Part model, mm, in its own coordinate system. A direction names the side the tool comes from. Give positions to 0.01 mm unless a question says otherwise; leave off trailing zeros. Write each loop counter-clockwise with the first axis right and the second up, starting at its lowest first coordinate (ties: lowest second). Pieces come first, ordered by that corner, then holes. Notation, with made-up numbers: M -16.5,57.5 L 20.5,57.5 A32 ccw 20.5,87.5 Z; hole C 7.5,50 d7. An arc over 180 degrees is marked long. Answer as CSV lines item,"result". Start each with the question number.
Item 1: Pin check, flat tips, straight feed: pin 1 (2.5 mm diameter, centred on y = 3, z = 11, fed in from -X); pin 2 (5 mm diameter, centred on x = -17.5, z = 24, fed in from +Y); pin 3 (1.5 mm diameter, centred on y = 18, z = 27.5, fed in from +X). Stop position of each tip, or through.
Item 2: Wall check: L1, parallel to Y at x = -9.25, z = 26.5; L2, parallel to X at y = 10, z = 28.5. Give the ranges that are in metal, low to high. Write a range as from..to.
Item 3: 3-axis set-ups, long thin cutter, end or side, ignore diameter. For faces 1 (the flat face through (-23, 30, 27)), 2 (the flat face through (-21, 8, 25)), 3 (the flat face through (-20, 17, 27)): which of +Z, -Z, +X, -X, +Y, -Y reach the whole face in a straight line?
Item 4: Band-saw the part on B-B, the plane z = 14. List the corners of the cut face in (x, y).
Item 5: Band-saw the part on C-C, the plane x = -4.5. List the corners of the cut face in (y, z).
Item 6: Band-saw the part on A-A, the plane y = 4. List the corners of the cut face in (x, z), then the cut area to 3 significant figures.
Autodesk Inventor part; units mm, degrees
ref_plane "YZ Plane" through (0, 0, 0) normal (1, 0, 0) x (0, 1, 0)
ref_plane "XZ Plane" through (0, 0, 0) normal (0, 1, 0) x (-1, 0, 0)
ref_plane "XY Plane" through (0, 0, 0) normal (0, 0, 1) x (1, 0, 0)
sketch "草圖1" plane through (0, 0, 0) normal (0, 0, 1) x (1, 0, 0)
  line L0 (0, 0) -> (5, 0)
  line L1 (5, 0) -> (5, 5)
  line L2 (5, 5) -> (0, 5)
  line L3 (0, 5) -> (0, 0)
  dimension "d0" = 5
  dimension "d1" = 5
extrude "擠出1" add sketch "草圖1" along normal blind 30
sketch "草圖2" plane through (0, 0, 0) normal (-1, 0, 0) x (0, 0, 1)
  line L0 (30, 0) -> (30, 5)
  line L1 (0, 0) -> (30, 0)
  line L2 (30, 5) -> (25, 5)
  line L3 (25, 5) -> (25, 0)
  line L4 (25, 0) -> (30, 0)
  line L5 (30, 0) -> (30, 5)
  dimension "d4" = 5
extrude "擠出2" add sketch "草圖2" along normal blind 25
sketch "草圖3" plane through (0, 5, 0) normal (0, 1, 0) x (1, 0, 0)
  line L0 (-25, -30) -> (-25, -25)
  line L1 (5, -30) -> (-25, -30)
  line L2 (-25, -25) -> (-20, -25)
  line L3 (-20, -25) -> (-20, -30)
  line L4 (-20, -30) -> (-25, -30)
  line L5 (-25, -30) -> (-25, -25)
  point P0 (0, 0)
  dimension "d7" = 5
extrude "擠出3" add sketch "草圖3" along normal blind 25
sketch "草圖4" plane through (0, 0, 0) normal (0, -1, 0) x (1, 0, 0)
  line L0 (5, 0) -> (0, 5)
  line L1 (5, 5) -> (0, 10)
  dimension "d11" = 5
sketch "草圖5" plane through (5, 0, 0) normal (1, 0, 0) x (0, 0, -1)
  line L0 (0, 0) -> (0, 5)
  line L1 (0, 0) -> (-30, 0)
  line L2 (0, 5) -> (-5, 5)
  line L3 (-5, 5) -> (-5, 0)
  line L4 (-5, 0) -> (0, 0)
  line L5 (0, 0) -> (0, 5)
  dimension "d10" = 5
properties part number "triangle"
Output:
1,pin 1,"x = 0"
1,pin 2,"y = 5"
1,pin 3,"x = -20"
2,L1,"0..5"
2,L2,"-25..-20"
3,face 1,"+Z, -Z, +X, -X, +Y"
3,face 2,"-Z, -X, +Y, -Y"
3,face 3,"+Z, -Z, +X, +Y"
4,outline,"M 0,0 L 5,0 L 5,5 L 0,5 Z"
5,outline,"M 0,25 L 5,25 L 5,30 L 0,30 Z"
6,outline,"M -25,25 L 0,25 L 0,0 L 5,0 L 5,30 L -25,30 Z"
6,area,"275 mm²"
